Input: part model. Units: mm. Frame: model coordinates. Face numbers are marked on the shaded views. A direction names the side the tool comes from. Give positions to 0.01 mm unless a question says otherwise; leave off trailing zeros. Order: outer loops, then holes, each group sorted by start corner. A loop starts at its lowest first (then second) coordinate and runs counter-clockwise, first axis right, second up.
Autodesk Inventor part; units mm, degrees
ref_plane "YZ Plane" through (0, 0, 0) normal (1, 0, 0) x (0, 1, 0)
ref_plane "XZ Plane" through (0, 0, 0) normal (0, 1, 0) x (-1, 0, 0)
ref_plane "XY Plane" through (0, 0, 0) normal (0, 0, 1) x (1, 0, 0)
sketch "Sketch1" plane through (0, 0, 0) normal (0, 0, 1) x (1, 0, 0)
  line L0 (2.75, -2.75) -> (-2.75, -2.75)
  line L1 (-2.75, -2.75) -> (-2.75, 2.75)
  line L2 (-2.75, 2.75) -> (2.75, 2.75)
  line L3 (2.75, 2.75) -> (2.75, -2.75)
  line L4 (2.75, -2.75) -> (-2.75, 2.75) construction
  line L5 (-2.75, -2.75) -> (2.75, 2.75) construction
  line L6 (1, 0.25) -> (1, 5.25)
  line L7 (1, 5.25) -> (-1, 5.25)
  line L8 (-1, 5.25) -> (-1, 0.25)
  line L9 (-1, 0.25) -> (1, 0.25)
  line L10 (1, 0.25) -> (-1, 5.25) construction
  line L11 (1, 5.25) -> (-1, 0.25) construction
  point P0 (0, 0)
  point P1 (0, 2.75)
  point P2 (-1, 2.75)
  point P3 (1, 2.75)
  dimension "d0" = 5.5
  dimension "d1" = 5.5
  dimension "d2" = 2
  dimension "d3" = 5
extrude "Extrusion1" add sketch "Sketch1" along normal blind 5.5
properties part number "Agarose-block"
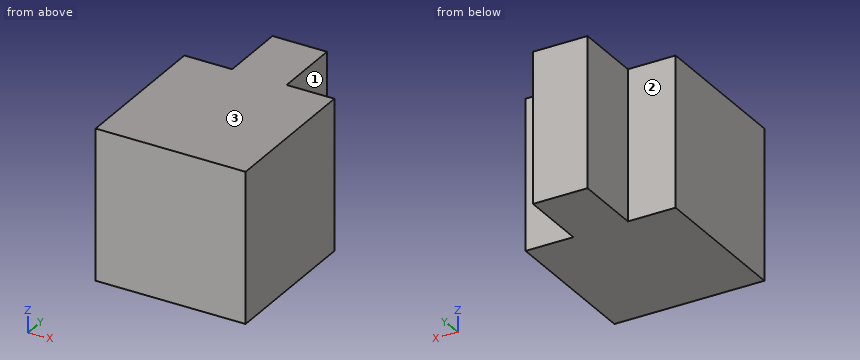
1) Cut plane B-B (x = 1.95). Return the cut outline in (y, z), then the cut area to 4 significant figures.
2) Cut plane A-A (z = 1.15). Return the cut outline in (x, y).
3) Reachability of the marked faces 1, 2 and 3 from +Z, -Z, +X, -X, +Y, -Y: full face, straight path, thin tool, end or side. Return the list, or none.
4) First-contact query: P1, Ø0.9, axis at x = -1.5, z = 2.5, coming from the +Y side; P2, Ø0.8, axis at y = 4.5, z = 2.5, coming from the -X side. Flat tips, straight axial feed; report the tip coordinate or a pass-through.
5) Line query: probe 1 along X at (y, z) = (4.25, 0.25); probe 2 along Y at (x, z) = (1.85, 4.9). Output: solid intervals per line, ascending.
Geometry says:
1. outline: (-2.75, 0) - (2.75, 0) - (2.75, 5.5) - (-2.75, 5.5) - close
1. area: 30.25 mm2
2. outline: (-2.75, -2.75) - (2.75, -2.75) - (2.75, 2.75) - (1, 2.75) - (1, 5.25) - (-1, 5.25) - (-1, 2.75) - (-2.75, 2.75) - close
3. face 1: +Z, -Z, +X, +Y
3. face 2: +Z, -Z, -X, +Y
3. face 3: +Z, +X, -X, +Y, -Y
4. P1: stops at y = 2.75
4. P2: stops at x = -1
5. probe 1: x = -1 to 1
5. probe 2: y = -2.75 to 2.75
